The model under review builds one solid part; all positions refer to its coordinate system, in mm. A direction names the side the tool comes from. Give positions to 0.01 mm unless a question says otherwise; leave off trailing zeros. Order: outer loops, then holes, each group sorted by start corner. A loop starts at its lowest first (then second) coordinate and runs counter-clockwise, first axis right, second up.
```python
from build123d import *

# Parameters (mm, degrees)
SKETCH1_W               = 36
SKETCH1_H               = 100
BOSS_EXTRUDE1_DEPTH     = 100
CUT_EXTRUDE1_DEPTH      = 118.45637488
CUT_EXTRUDE1_DEPTH_BACK = 118.45637488
CUT_EXTRUDE5_DEPTH      = 118.45637488
CUT_EXTRUDE5_DEPTH_BACK = 118.45637488
FILLET3_R               = 4
CUT_EXTRUDE6_DEPTH      = 107.244999882
CUT_EXTRUDE6_DEPTH_BACK = 107.244999882
SKETCH9_R               = 4
CUT_EXTRUDE7_DEPTH      = 138.069325525
CUT_EXTRUDE7_DEPTH_BACK = 138.069325525
SKETCH10_R              = 4


with BuildPart() as part:
    # Sketch1 → Boss-Extrude1 (new body)
    with BuildSketch(Plane(origin=(0, 0, 0), x_dir=(1, 0, 0), z_dir=(0, 1, 0))):
        Rectangle(SKETCH1_W, SKETCH1_H)
    extrude(amount=BOSS_EXTRUDE1_DEPTH)

    # Sketch2 → Cut-Extrude1 (cut, two sides: drawn at the far end of the back side and taken through both)
    with BuildSketch(Plane.ZY.offset(18).offset(-CUT_EXTRUDE1_DEPTH_BACK)):
        Polygon((50, 100), (-42, 100), (-42, 64), (14, 8), (50, 8), align=None)
    extrude(amount=CUT_EXTRUDE1_DEPTH + CUT_EXTRUDE1_DEPTH_BACK, mode=Mode.SUBTRACT)

    # Sketch8 → Cut-Extrude5 (cut, two sides: drawn at the far end of the back side and taken through both)
    with BuildSketch(Plane(origin=(18, 0, 0), x_dir=(0, 0, -1), z_dir=(1, 0, 0)).offset(-CUT_EXTRUDE5_DEPTH_BACK)):
        with BuildLine():
            Line((42, 43.029437252), (42, 12))
            ThreePointArc((42, 12), (40.828427125, 9.171572875), (38, 8))
            Line((38, 8), (6.970562748, 8))
            ThreePointArc((6.970562748, 8), (3.275044618, 10.469266271), (4.142135624, 14.828427125))
            Line((4.142135624, 14.828427125), (35.171572875, 45.857864376))
            ThreePointArc((35.171572875, 45.857864376), (39.530733729, 46.724955382), (42, 43.029437252))
        make_face()
    extrude(amount=CUT_EXTRUDE5_DEPTH + CUT_EXTRUDE5_DEPTH_BACK, mode=Mode.SUBTRACT)

    # Fillet3
    fillet3_edges = [part.edges().sort_by_distance(p)[0] for p in [
        (-18, 100, -46),
        (18, 100, -46),
        (18, 4, 50),
        (-18, 4, 50),
        (0, 0, -50),
    ]]
    fillet(fillet3_edges, radius=FILLET3_R)

    # Sketch9 → Cut-Extrude6 (cut, two sides: drawn at the far end of the back side and taken through both)
    with BuildSketch(Plane(origin=(0, 8, 0), x_dir=(1, 0, 0), z_dir=(0, 1, 0)).offset(-CUT_EXTRUDE6_DEPTH_BACK)):
        with Locations(Location((0, -30, 0), (0, 0, 270))):
            Circle(SKETCH9_R)
    extrude(amount=CUT_EXTRUDE6_DEPTH + CUT_EXTRUDE6_DEPTH_BACK, mode=Mode.SUBTRACT)

    # Sketch10 → Cut-Extrude7 (cut, two sides: drawn at the far end of the back side and taken through both)
    with BuildSketch(Plane.XY.offset(-42).offset(-CUT_EXTRUDE7_DEPTH_BACK)):
        with Locations((0, 80)):
            Circle(SKETCH10_R)
    extrude(amount=CUT_EXTRUDE7_DEPTH + CUT_EXTRUDE7_DEPTH_BACK, mode=Mode.SUBTRACT)


solid = part.part
```
Item 1: Take a section at C-C (y = 40). Give the boundary of the cut face in (x, z).
Values found:
outline: (-18, -50) - (18, -50) - (18, -42) - (-18, -42) - close; (-18, -29.31) - (18, -29.31) - (18, -18) - (-18, -18) - close
Item 2: Take a section at A-A (x = 0). Give the boundary of the cut face in (y, z), and give its area (3 significant figures).
Values found:
outline: (0, -46) arc R4 ccw to (4, -50) - (76, -50) - (76, -42) - (64, -42) - (8, 14) - (8, 26) - (0, 26) - close; (0, 34) - (8, 34) - (8, 50) - (0, 50) - close; (84, -50) - (100, -50) - (100, -42) - (84, -42) - close; hole (8, -38) arc R4 ccw to (12, -42) - (43.03, -42) arc R4 ccw to (45.86, -35.17) - (14.83, -4.14) arc R4 ccw to (8, -6.97) - close
area: 2,020 mm2
Item 3: For faces 1 (the flat face through (0, 100, -46)), 2 (the flat face through (0, 8, -23)), 3 (the flat face through (0, 86, -42)), list the 3-axis set-ups (+Z, -Z, +X, -X, +Y, -Y) from which the entire face can be reached by the end or side of a thin tool; tool diameter is ignored.
Values found:
face 1: +Z, -Z, +X, -X, +Y
face 2: +X, -X
face 3: +Z, +X, -X, +Y
Item 4: Draft analysis for pull direction X (two halves, no side actions). For faces 4 (the cylindrical face through (16.797, 4.056, 48.859)), 5 (the cylindrical face through (-16.859, 4.056, 48.797)), 6 (the cylindrical face through (-0.25, 46.75, -39.47)), 7 (the cylindrical face through (-2.4, 3.9, 26.8)), state which applies: released by +X, released by -X, zero draft, split by the parting line, or undercut.
Values found:
face 4: released by +X
face 5: released by -X
face 6: zero draft
face 7: undercut
Item 5: For line 1 (Z direction, x = 0, y = 4.75); line 2 (Y direction, x = 0, z = -45.5); line 3 (X direction, y = 80, z = -44), list the stretches that pass through material, from the lowest coordinate up.
Values found:
line 1: z = -50 to 26, 34 to 50
line 2: y = 0 to 76, 84 to 100
line 3: x = -18 to -4, 4 to 18
Item 6: Take a section at B-B (z = 30). Give the boundary of the cut face in (x, y), and give its area (3 significant figures).
Values found:
outline: (-18, 0) - (-4, 0) - (-4, 8) - (-18, 8) - close; (4, 0) - (18, 0) - (18, 8) - (4, 8) - close
area: 224 mm2
Item 7: Clearance check with flat-ended pins moving along their axes: pin 1 Ø1 at (x, y) = (-6.5, 51.5) entering from +Z; pin 2 Ø4 at (x, y) = (0.5, 64) entering from +Z; pin 3 Ø11 at (x, y) = (-5, 84.5) entering from +Z. State where each tip first meets the part, or that it passes through.
Values found:
pin 1: stops at z = -29
pin 2: stops at z = -40
pin 3: stops at z = -42
Item 8: Take a section at D-D (x = 5.5). Give the boundary of the cut face in (y, z).
Values found:
outline: (0, -46) arc R4 ccw to (4, -50) - (100, -50) - (100, -42) - (64, -42) - (8, 14) - (8, 50) - (0, 50) - close; hole (8, -38) arc R4 ccw to (12, -42) - (43.03, -42) arc R4 ccw to (45.86, -35.17) - (14.83, -4.14) arc R4 ccw to (8, -6.97) - close
